from build123d import *

# Parameters (mm, degrees)
F0_W     = 30
F0_H     = 15
F1_DEPTH = 4
F2_R     = 3
F3_DEPTH = 25
F4_ANGLE = 45


with BuildPart() as f1:
    # F0 (on Top) → F1 (new body)
    with BuildSketch(Plane.XY):
        Rectangle(F0_W, F0_H)
    extrude(amount=F1_DEPTH)


with BuildPart() as f3:
    # F2 (on Top) → F3 (new body)
    with BuildSketch(Plane.XY):
        with Locations((0, -2.5)):
            Circle(F2_R)
    extrude(amount=F3_DEPTH)


with BuildPart() as f3_1:
    # F4: moved
    add(f3.part.rotate(Axis((0, -7.5, 4), (-1, 0, 0)), F4_ANGLE))


with BuildPart() as f3_2:
    # F5: moved
    add(f3_1.part.moved(Location((0, 2, 6.25))))


with BuildPart() as f1_1:
    add(f1.part)

    # F6: cut F3
    add(f3_2.part, mode=Mode.SUBTRACT)


solid = f1_1.part
Source: CAD feature listing. Evaluate the final solid. Frame: model axes, mm. A direction names the side the tool comes from. Coordinates: 2 decimals unless noted, no trailing zeros. Answer in a Markdown table with one row per item.
Q1. Set-up query: faces 4 (the flat face through (-0.042, -4.022, 3.115)), 5 (the flat face through (-15, 0, 2)). Return all of +Z, -Z, +X, -X, +Y, -Y with unobstructed straight access to the full face (end or side cutting, diameter ignored); none if empty.
Answers below:
| item | result |
|---|---|
| face 4 | +Z |
| face 5 | +Z, -Z, -X, +Y, -Y |
Q2. Draft query along Y for faces 1 (the cylindrical face through (0.068, -1.814, 2.623)), 2 (the flat face through (15, 0, 2)), 3 (the flat face through (0, 7.5, 2)). Return one class per face: pulls with the +Y half, pulls with the -Y half, needs draft (parallel to the pull), parting line crosses it, or undercut.
Answers below:
| item | result |
|---|---|
| face 1 | undercut |
| face 2 | needs draft |
| face 3 | pulls with the +Y half |
Q3. Ray query, probe 1 along Z at (x, y) = (-0.25, -2). Return the intervals inside material, ascending. Write a range as from..to.
Answers below:
| item | result |
|---|---|
| probe 1 | z = 0..2.45 |
